from build123d import *

# Parameters (mm, degrees)
PAD001_DEPTH    = 30
PAD_DEPTH       = 15
SKETCH001_R     = 13.5
POCKET_DEPTH    = 3
SKETCH003_R     = 5.1
SKETCH003_R_2   = 1.1
POCKET001_DEPTH = 5


with BuildPart() as profile_pad:
    # Sketch002 → Pad001 (new body, symmetric)
    with BuildSketch(Plane.XZ):
        Polygon((19.421573, 10), (-17.25, 10), (-17.25, 15), (17.25, 15), (30.25, 2), (36.75, 2), (41.75, 0), (29.421573, 0), align=None)
    extrude(amount=PAD001_DEPTH, both=True)


with BuildPart() as holes:
    # Sketch → Pad (new body)
    with BuildSketch(Plane.XY):
        with BuildLine():
            ThreePointArc((0, 17.25), (-17.250031, 0), (0, -17.25))
            Line((0, -17.25), (17.25, -17.25))
            Line((17.25, -17.25), (27, -25))
            Line((27, -25), (47, -25))
            Line((47, -25), (47, 25))
            Line((47, 25), (27, 25))
            Line((17.25, 17.25), (27, 25))
            Line((17.25, 17.25), (0, 17.25))
        make_face()
    extrude(amount=PAD_DEPTH)

    # Common: intersect Profile Pad
    add(profile_pad.part, mode=Mode.INTERSECT)

    # Sketch001 → Pocket (cut)
    with BuildSketch(Plane.XY.offset(15)):
        Circle(SKETCH001_R)
    extrude(amount=-POCKET_DEPTH, mode=Mode.SUBTRACT)

    # Sketch003 → Pocket001 (cut)
    with BuildSketch(Plane.XY.offset(12)):
        Circle(SKETCH003_R)
        with Locations((-11.25, 0)):
            Circle(SKETCH003_R_2)
        with Locations((0, 11.25)):
            Circle(SKETCH003_R_2)
        with Locations((11.25, 0)):
            Circle(SKETCH003_R_2)
        with Locations((0, -11.25)):
            Circle(SKETCH003_R_2)
        with Locations((-5.625, 9.742786)):
            Circle(SKETCH003_R_2)
        with Locations((-9.742786, 5.625)):
            Circle(SKETCH003_R_2)
        with Locations((-9.742786, -5.625)):
            Circle(SKETCH003_R_2)
        with Locations((-5.625, -9.742786)):
            Circle(SKETCH003_R_2)
        with Locations((5.625, -9.742786)):
            Circle(SKETCH003_R_2)
        with Locations((9.742786, -5.625)):
            Circle(SKETCH003_R_2)
        with Locations((5.625, 9.742786)):
            Circle(SKETCH003_R_2)
        with Locations((9.742786, 5.625)):
            Circle(SKETCH003_R_2)
    extrude(amount=-POCKET001_DEPTH, mode=Mode.SUBTRACT)


solid = holes.part
Input: part model. Units: mm. Frame: model coordinates. A direction names the side the tool comes from. Give positions to 0.01 mm unless a question says otherwise; leave off trailing zeros. Write each loop counter-clockwise with the first axis right and the second up, starting at its lowest first coordinate (ties: lowest second). Pieces come first, ordered by that corner, then holes. Notation, with made-up numbers: M 4.5,55 L 20.5,55 A19 ccw 20.5,87 Z; hole C 31.25,-24.5 d6. An arc over 180 degrees is marked long. Use one line per item in the form item = value.
1. Reachability of faces 1 (the face through (6, 0, 12)), 2 (the face through (9, -17.25, 12)), 3 (the face through (9, 17.25, 12)) from +Z, -Z, +X, -X, +Y, -Y: full face, straight path, thin tool, end or side. Return the list, or none.
Outcome:
face_1 = +Z
face_2 = +Z, -Z, -X, -Y
face_3 = +Z, -Z, -X, +Y
2. Ray query, L1, parallel to Y at x = 0, z = 11.05; L2, parallel to Z at x = -9, y = 3.5; L3, parallel to Z at x = 36, y = -15. Return the intervals inside material, ascending.
Outcome:
L1 = -17.25 to -12.35, -10.15 to -5.1, 5.1 to 10.15, 12.35 to 17.25
L2 = 10 to 12
L3 = 0 to 2
3. Mould query, pull axis Y, two halves, no side actions, for faces 4 (the face through (-10.55, -4.88, 11.01)), 5 (the face through (32.7, -25, 1.6)), 6 (the face through (33, 0, 2)). Classes: released by +Y, released by -Y, zero draft, split by the parting line, or undercut.
Outcome:
face_4 = undercut
face_5 = released by -Y
face_6 = zero draft
4. Cut plane B-B on y = -2.5. Return loops of the section in (x, z), and give its area (3 significant figures).
Outcome:
outline = M -17.07,10 L -4.45,10 L -4.45,12 L -13.27,12 L -13.27,15 L -17.07,15 Z; M 4.45,10 L 19.42,10 L 29.42,0 L 41.75,0 L 36.75,2 L 30.25,2 L 17.25,15 L 13.27,15 L 13.27,12 L 4.45,12 Z
area = 131 mm²
5. Cut plane A-A on y = -8. Return loops of the section in (x, z).
Outcome:
outline = M -15.28,10 L 19.42,10 L 29.42,0 L 41.75,0 L 36.75,2 L 30.25,2 L 17.25,15 L 10.87,15 L 10.87,12 L -10.87,12 L -10.87,15 L -15.28,15 Z
6. Cut plane D-D on x = 18.5. Return loops of the section in (y, z).
Outcome:
outline = M -18.24,10 L 18.24,10 L 18.24,13.75 L -18.24,13.75 Z
7. Cut plane C-C on z = 3.5. Return loops of the section in (x, y), and give its area (3 significant figures).
Outcome:
outline = M 25.92,-24.14 L 27,-25 L 28.75,-25 L 28.75,25 L 27,25 L 25.92,24.14 Z
area = 140 mm²
8. First-contact query: P1, Ø8, axis at x = -6.5, y = 4, coming from the +Z side; P2, Ø2, axis at x = 21.5, y = -12, coming from the -Z side; P3, Ø1.8, axis at x = 5.62, y = 9.74, coming from the -Z side; P4, Ø8, axis at y = 11.5, z = 11.5, coming from the -X side. Flat tips, straight axial feed; report the tip coordinate or a pass-through.
Outcome:
P1 = 12
P2 = 6.92
P3 = through
P4 = -15.53
